Part model, mm, in its own coordinate system. A direction names the side the tool comes from. Round coordinates to 2 decimals unless told otherwise and drop trailing zeros. Loops run counter-clockwise (first coordinate to the right, second up) from the corner with the lowest first, then second, coordinate; pieces in that order, holes last. Notation, with made-up numbers: (86.5, -7) - (140.5, -7) arc R5 cw to (140.5, 1) - close; hole circle Ø1 at (3.5, -1). An arc over 180 degrees is marked (long way). Put each result on its own line as item: value.
from build123d import *

# Parameters (mm, degrees)
Y_KSEKLIK_EKSTR_ZYON1_DEPTH      = 2
Y_KSEKLIK_EKSTR_ZYON1_DEPTH_BACK = 30
IZIM1_R                          = 12.470765814
Y_KSEKLIK_EKSTR_ZYON2_DEPTH      = 4.5
Y_KSEKLIK_EKSTR_ZYON2_DEPTH_BACK = 30
IZIM1_3_R                        = 12.470765814
IZIM1_3_R_2                      = 10.392304845
Y_KSEKLIK_EKSTR_ZYON3_DEPTH      = 2
Y_KSEKLIK_EKSTR_ZYON3_DEPTH_BACK = 30
IZIM1_4_R                        = 10.392304845
IZIM4_W                          = 3.2
IZIM4_H                          = 20
KES_EKSTR_ZYON1_DEPTH            = 5
DAIRESEL_KAPLAMA1_COUNT          = 3
IZIM6_R                          = 6
IZIM5_R                          = 4


with BuildPart() as part:
    # Çizim1 → Yükseklik-Ekstrüzyon1 (new, two sides: drawn at the far end of the back side and taken through both)
    with BuildSketch(Plane.XY.offset(-Y_KSEKLIK_EKSTR_ZYON1_DEPTH_BACK)):
        Polygon((-23.880099845, 2.396003215), (-14.015049574, -19.482771503), (9.86505027, -21.878774718), (23.880099845, -2.396003215), (14.015049574, 19.482771503), (-9.86505027, 21.878774718), align=None)
        Circle(IZIM1_R, mode=Mode.SUBTRACT)
    extrude(amount=Y_KSEKLIK_EKSTR_ZYON1_DEPTH + Y_KSEKLIK_EKSTR_ZYON1_DEPTH_BACK)

    # Çizim1<3> → Yükseklik-Ekstrüzyon2 (add, two sides: drawn at the far end of the back side and taken through both)
    with BuildSketch(Plane.XY.offset(-Y_KSEKLIK_EKSTR_ZYON2_DEPTH_BACK)):
        Circle(IZIM1_3_R)
        Circle(IZIM1_3_R_2, mode=Mode.SUBTRACT)
    extrude(amount=Y_KSEKLIK_EKSTR_ZYON2_DEPTH + Y_KSEKLIK_EKSTR_ZYON2_DEPTH_BACK)

    # Çizim1<4> → Yükseklik-Ekstrüzyon3 (add, two sides: drawn at the far end of the back side and taken through both)
    with BuildSketch(Plane.XY.offset(-Y_KSEKLIK_EKSTR_ZYON3_DEPTH_BACK)):
        Circle(IZIM1_4_R)
    extrude(amount=Y_KSEKLIK_EKSTR_ZYON3_DEPTH + Y_KSEKLIK_EKSTR_ZYON3_DEPTH_BACK)

    # Çizim4 → Kes-Ekstrüzyon1 (cut)
    with BuildSketch(Plane(origin=(16.872575058, -12.137388967, 0), x_dir=(0, 0, -1), z_dir=(0.8117821459477176, -0.5839603989317416, 0))):
        with Locations((2.622089109, 0)):
            Rectangle(IZIM4_W, IZIM4_H)
    kes_ekstr_zyon1 = extrude(amount=-KES_EKSTR_ZYON1_DEPTH, mode=Mode.SUBTRACT)

    # Dairesel Kaplama1: Kes-Ekstrüzyon1 ×3 about axis
    dairesel_kaplama1_axis = Axis((0, 0, 0), (0, 0, 1))
    for i in range(1, DAIRESEL_KAPLAMA1_COUNT):
        add(kes_ekstr_zyon1.rotate(dairesel_kaplama1_axis, i * 360 / DAIRESEL_KAPLAMA1_COUNT), mode=Mode.SUBTRACT)

    # Çizim6 → Loft1 section 0
    with BuildSketch(Plane(origin=(0, 0, -41), x_dir=(-1, 0, 0), z_dir=(0, 0, -1))):
        Circle(IZIM6_R)
    # Çizim5 → Loft1 section 1
    with BuildSketch(Plane(origin=(0, 0, -30), x_dir=(-1, 0, 0), z_dir=(0, 0, -1))):
        Circle(IZIM5_R)
    loft()


solid = part.part
1. Band-saw the part on C-C (x = -7). List the corners of the cut face in (y, z), plus the area to 3 significant figures.
A:
outline: (-20.19, -30) - (21.59, -30) - (21.59, -4.22) - (16.57, -4.22) - (16.57, -1.02) - (21.59, -1.02) - (21.59, 2) - (10.32, 2) - (10.32, 4.5) - (7.68, 4.5) - (7.68, 2) - (-7.68, 2) - (-7.68, 4.5) - (-10.32, 4.5) - (-10.32, 2) - (-20.19, 2) - close
area: 1,330 mm²
2. Two-plate mould, pull along Z, no slides. Class faces 6 (the flat face through (2, 18, -4.222)), 7 (the flat face through (0, 0, 2)), 8 (the flat face through (-16.774, 12.274, -14.224)): pulls with the +Z half, pulls with the -Z half, needs draft (parallel to the pull), parting line crosses it, or undercut.
A:
face 6: undercut
face 7: pulls with the +Z half
face 8: needs draft
3. Tool access for faces 1 (the flat face through (2.242, 20.664, -14.224)), 2 (the flat face through (9.032, -18.816, -2.6)), 3 (the flat face through (12.9, -9.1, -2.6)), 4 (the flat face through (0, 0, -41)), 5 (the flat face through (10, 10, 2)): list every direction of +Z, -Z, +X, -X, +Y, -Y with a clear straight run to the whole face (end or side of a thin tool).
A:
face 1: +Z, -Z, +X, +Y
face 2: +X
face 3: none
face 4: -Z, +X, -X, +Y, -Y
face 5: +Z
4. Pin check, flat tips, straight feed: P1, Ø5, axis at x = -14, z = -1, coming from the -Y side; P2, Ø10, axis at x = -17.5, y = -9.5, coming from the +Z side; P3, Ø10, axis at x = 0.5, y = -11.5, coming from the -Z side. Stop position of each tip, or through.
A:
P1: stops at y = -19.74
P2: stops at z = 2
P3: stops at z = -30
5. Band-saw the part on A-A (z = 1). List the corners of the cut face in (x, y).
A:
outline: (-23.88, 2.4) - (-14.02, -19.48) - (9.87, -21.88) - (23.88, -2.4) - (14.02, 19.48) - (-9.87, 21.88) - close
6. Probe line 1 along Z through (x, y) = (-13.5, -12); line 2 along Y through (x, z) = (0, 3.15); line 3 along Z through (x, y) = (-11, 19.5). List the from-to ranges inside material, lowest first. Write a range as [from, to].
A:
line 1: z = [-30, -4.22], [-1.02, 2]
line 2: y = [-12.47, -10.39], [10.39, 12.47]
line 3: z = [-30, 2]
7. Band-saw the part on B-B (x = 0). List the corners of the cut face in (y, z).
A:
outline: (-20.89, -30) - (-4, -30) - (-6, -41) - (6, -41) - (4, -30) - (20.89, -30) - (20.89, -4.22) - (15.86, -4.22) - (15.86, -1.02) - (20.89, -1.02) - (20.89, 2) - (12.47, 2) - (12.47, 4.5) - (10.39, 4.5) - (10.39, 2) - (-10.39, 2) - (-10.39, 4.5) - (-12.47, 4.5) - (-12.47, 2) - (-20.89, 2) - close
